```python
from build123d import *
from OCP.BRepFilletAPI import BRepFilletAPI_MakeChamfer

# Parameters (mm, degrees)
SKETCH1_W                   = 61.468
SKETCH1_H                   = 29.21
BOSS_EXTRUDE1_DEPTH         = 0.762
F_32_0_116_DIAMETER_HOLE1_D = 2.9464
SKETCH4_W                   = 10.16
SKETCH4_H                   = 10.16
BOSS_EXTRUDE2_DEPTH         = 13.97
SKETCH5_W                   = 10.16
SKETCH5_H                   = 10.16
BOSS_EXTRUDE3_DEPTH         = 13.97
CHAMFER1_SIZE               = 6.35
CHAMFER1_SIZE2              = 1.701477372
SKETCH6_R                   = 2.3495
BOSS_EXTRUDE4_DEPTH         = 12.7
SKETCH7_W                   = 21.517957465
SKETCH7_H                   = 14.561058099
BOSS_EXTRUDE5_DEPTH         = 15.875
SKETCH8_R                   = 2.468766422
BOSS_EXTRUDE6_DEPTH         = 12.7


with BuildPart() as part:
    # Sketch1 → Boss-Extrude1 (new, symmetric)
    with BuildSketch(Plane(origin=(0, 0, 0), x_dir=(1, 0, 0), z_dir=(0, 1, 0))):
        Rectangle(SKETCH1_W, SKETCH1_H)
    extrude(amount=BOSS_EXTRUDE1_DEPTH, both=True)

    # #32 (0.116) Diameter Hole1 (through all)
    with Locations(Plane(origin=(0, 0.762, 0), x_dir=(1, 0, 0), z_dir=(0, 1, 0))):
        with Locations((-27.686, 11.303), (-27.686, -11.303)):
            Hole(F_32_0_116_DIAMETER_HOLE1_D / 2)

    # Sketch4 → Boss-Extrude2 (add)
    with BuildSketch(Plane(origin=(0, 0.762, 0), x_dir=(1, 0, 0), z_dir=(0, 1, 0))):
        with Locations((-25.146, 0)):
            Rectangle(SKETCH4_W, SKETCH4_H)
    extrude(amount=BOSS_EXTRUDE2_DEPTH)

    # Sketch5 → Boss-Extrude3 (add)
    with BuildSketch(Plane(origin=(0, 0.762, 0), x_dir=(1, 0, 0), z_dir=(0, 1, 0))):
        with Locations((25.146, 7.493)):
            Rectangle(SKETCH5_W, SKETCH5_H)
        with Locations((25.146, -7.493)):
            Rectangle(SKETCH5_W, SKETCH5_H)
    extrude(amount=BOSS_EXTRUDE3_DEPTH)

    # Chamfer1: one chamfer whose edges measure the first distance from different faces: ONE call of the kernel's chamfer builder (chamfer() names one face for all edges)
    chamfer1_edges_1 = [part.edges().sort_by_distance(p)[0] for p in [
        (-30.226, 14.732, 0),
    ]]
    chamfer1_side_1 = [part.faces().sort_by_distance(p)[0] for p in [
        (-30.226, 7.747, 0),
    ]]
    chamfer1_edges_2 = [part.edges().sort_by_distance(p)[0] for p in [
        (-20.066, 14.732, 0),
    ]]
    chamfer1_side_2 = [part.faces().sort_by_distance(p)[0] for p in [
        (-20.066, 7.747, 0),
    ]]
    chamfer1_edges_3 = [part.edges().sort_by_distance(p)[0] for p in [
        (20.066, 14.732, -7.493),
    ]]
    chamfer1_side_3 = [part.faces().sort_by_distance(p)[0] for p in [
        (20.066, 7.747, -7.493),
    ]]
    chamfer1_edges_4 = [part.edges().sort_by_distance(p)[0] for p in [
        (30.226, 14.732, -7.493),
    ]]
    chamfer1_side_4 = [part.faces().sort_by_distance(p)[0] for p in [
        (30.226, 7.747, -7.493),
    ]]
    chamfer1_edges_5 = [part.edges().sort_by_distance(p)[0] for p in [
        (20.066, 14.732, 7.493),
    ]]
    chamfer1_side_5 = [part.faces().sort_by_distance(p)[0] for p in [
        (20.066, 7.747, 7.493),
    ]]
    chamfer1_edges_6 = [part.edges().sort_by_distance(p)[0] for p in [
        (30.226, 14.732, 7.493),
    ]]
    chamfer1_side_6 = [part.faces().sort_by_distance(p)[0] for p in [
        (30.226, 7.747, 7.493),
    ]]
    chamfer1 = BRepFilletAPI_MakeChamfer(part.part.solid().wrapped)
    for e in chamfer1_edges_1:
        chamfer1.Add(CHAMFER1_SIZE, CHAMFER1_SIZE2, e.wrapped, chamfer1_side_1[0].wrapped)  # the first distance lies on this face
    for e in chamfer1_edges_2:
        chamfer1.Add(CHAMFER1_SIZE, CHAMFER1_SIZE2, e.wrapped, chamfer1_side_2[0].wrapped)  # the first distance lies on this face
    for e in chamfer1_edges_3:
        chamfer1.Add(CHAMFER1_SIZE, CHAMFER1_SIZE2, e.wrapped, chamfer1_side_3[0].wrapped)  # the first distance lies on this face
    for e in chamfer1_edges_4:
        chamfer1.Add(CHAMFER1_SIZE, CHAMFER1_SIZE2, e.wrapped, chamfer1_side_4[0].wrapped)  # the first distance lies on this face
    for e in chamfer1_edges_5:
        chamfer1.Add(CHAMFER1_SIZE, CHAMFER1_SIZE2, e.wrapped, chamfer1_side_5[0].wrapped)  # the first distance lies on this face
    for e in chamfer1_edges_6:
        chamfer1.Add(CHAMFER1_SIZE, CHAMFER1_SIZE2, e.wrapped, chamfer1_side_6[0].wrapped)  # the first distance lies on this face
    add(Compound.cast(chamfer1.Shape()), mode=Mode.REPLACE)

    # Sketch6 → Boss-Extrude4 (add)
    with BuildSketch(Plane(origin=(0, 0.762, 0), x_dir=(1, 0, 0), z_dir=(0, 1, 0))):
        with Locations(Location((-20.420225117, 10.051406146, 0), (0, 0, 270))):
            Circle(SKETCH6_R)
    extrude(amount=BOSS_EXTRUDE4_DEPTH)

    # Sketch7 → Boss-Extrude5 (add)
    with BuildSketch(Plane(origin=(0, 0.762, 0), x_dir=(1, 0, 0), z_dir=(0, 1, 0))):
        with Locations((-0.009722788, 2.057247528)):
            Rectangle(SKETCH7_W, SKETCH7_H)
    extrude(amount=BOSS_EXTRUDE5_DEPTH)

    # Sketch8 → Boss-Extrude6 (add)
    with BuildSketch(Plane(origin=(0, 0.762, 0), x_dir=(1, 0, 0), z_dir=(0, 1, 0))):
        with Locations(Location((2.574570697, -7.864784458, 0), (0, 0, 270))):
            Circle(SKETCH8_R)
    extrude(amount=BOSS_EXTRUDE6_DEPTH)


solid = part.part
```
Input: part model. Units: mm. Frame: model coordinates. A direction names the side the tool comes from. Give positions to 0.01 mm unless a question says otherwise; leave off trailing zeros. Order: outer loops, then holes, each group sorted by start corner. A loop starts at its lowest first (then second) coordinate and runs counter-clockwise, first axis right, second up.
1. Cut plane D-D (x = 10). Return loops of the section in (y, z) (3 decimals), and give its area (3 significant figures).
Computed:
outline: (-0.762, -14.605) - (0.762, -14.605) - (0.762, -9.338) - (16.637, -9.338) - (16.637, 5.223) - (0.762, 5.223) - (0.762, 14.605) - (-0.762, 14.605) - close
area: 276 mm2
2. Line query: probe 1 along X at (y, z) = (5.5, 2.75); probe 2 along Z at (x, y) = (27, 11); probe 3 along Z at (x, y) = (2.5, 1.5). Output: solid intervals per line, ascending.
Computed:
probe 1: x = -30.23 to -20.07, -10.77 to 10.75, 20.07 to 30.23
probe 2: z = -12.57 to -2.41, 2.41 to 12.57
probe 3: z = -9.34 to 5.22, 5.4 to 10.33
3. Cut plane A-A (x = 24). Return loops of the section in (y, z) (3 decimals), and give its area (3 significant figures).
Computed:
outline: (-0.762, -14.605) - (0.762, -14.605) - (0.762, -12.573) - (14.732, -12.573) - (14.732, -2.413) - (0.762, -2.413) - (0.762, 2.413) - (14.732, 2.413) - (14.732, 12.573) - (0.762, 12.573) - (0.762, 14.605) - (-0.762, 14.605) - close
area: 328 mm2
4. Set-up query: faces 1 (the face through (10.749, 9, -2)), 2 (the face through (-20.066, 5, 0)), 3 (the face through (25, 8, -2.413)), 4 (the face through (-30.226, 5, 0)). Return all of +Z, -Z, +X, -X, +Y, -Y with unobstructed straight access to the full face (end or side cutting, diameter ignored); none if empty.
Computed:
face 1: +Z, -Z, +Y
face 2: +Z, +Y
face 3: +X, +Y
face 4: +Z, -Z, -X, +Y
5. Draft query along Z for faces 5 (the face through (20.93, 11.6, -7.42)), 6 (the face through (25, 8, 12.573)), 7 (the face through (25, 8, 2.413)), 8 (the face through (0, 9, 5.223)). Return one class per face: released by +Z, released by -Z, zero draft, split by the parting line, or undercut.
Computed:
face 5: zero draft
face 6: released by +Z
face 7: undercut
face 8: undercut
6. Cut plane B-B (y = 11). Return loops of the section in (x, z).
Computed:
outline: (-29.52, -5.08) - (-20.77, -5.08) - (-20.77, 5.08) - (-29.52, 5.08) - close; circle Ø4.7 at (-20.42, -10.05); (-10.77, -9.34) - (10.75, -9.34) - (10.75, 5.22) - (-10.77, 5.22) - close; circle Ø4.94 at (2.57, 7.86); (20.77, -12.57) - (29.52, -12.57) - (29.52, -2.41) - (20.77, -2.41) - close; (20.77, 2.41) - (29.52, 2.41) - (29.52, 12.57) - (20.77, 12.57) - close
7. Pin query (flat end, axial travel): pin 1 Ø2 at (x, z) = (24.5, 9) entering from +Y; pin 2 Ø5 at (x, y) = (1.5, 10.5) entering from +Z; pin 3 Ø8 at (x, y) = (23, 6.5) entering from -Z. Return the tip coordinate at first contact, or that it passes through.
Computed:
pin 1: stops at y = 14.73
pin 2: stops at z = 10.33
pin 3: stops at z = -12.57
8. Cut plane C-C (z = -1.75). Return loops of the section in (x, y), and give its area (3 significant figures).
Computed:
outline: (-30.73, -0.76) - (30.73, -0.76) - (30.73, 0.76) - (10.75, 0.76) - (10.75, 16.64) - (-10.77, 16.64) - (-10.77, 0.76) - (-20.07, 0.76) - (-20.07, 8.38) - (-21.77, 14.73) - (-28.52, 14.73) - (-30.23, 8.38) - (-30.23, 0.76) - (-30.73, 0.76) - close
area: 566 mm2
